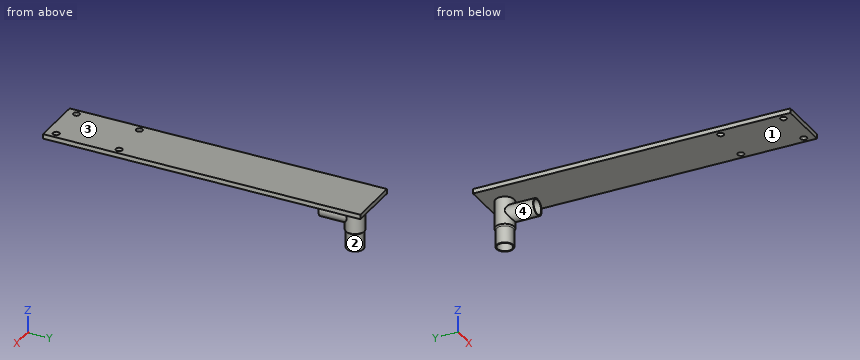
```python
from build123d import *

# Parameters (mm, degrees)
SKETCH_1_W             = 56
SKETCH_1_H             = 89.4
EXTRUDE_1_DEPTH        = 5
HOLE_WIZARD_M8_2_D     = 6.8
HOLE_WIZARD_M8_2_DEPTH = 19.75
HOLE_WIZARD_M8_2_TIP   = 2.042926105
SKETCH_7_W             = 56
SKETCH_7_H             = 5
EXTRUDE_2_DEPTH        = 252.5709
SKETCH_8_R             = 10
EXTRUDE_3_DEPTH        = 30
SKETCH_9_R             = 9
EXTRUDE_4_DEPTH        = 20
FILLET_1_R             = 2
EXTRUDE_START          = -20
SKETCH_10_R            = 9
EXTRUDE_5_DEPTH        = 35
SKETCH_11_R            = 8
CUT_EXTRUDE_1_DEPTH    = 40
SKETCH_12_R            = 8
CUT_EXTRUDE_2_DEPTH    = 45


with BuildPart() as part:
    # 草图1 → 凸台-拉伸1 (new body)
    with BuildSketch(Plane.XY):
        with Locations((28, -44.7)):
            Rectangle(SKETCH_1_W, SKETCH_1_H)
    extrude(amount=EXTRUDE_1_DEPTH)

    # M8 螺纹孔2
    with Locations(Plane.XY.offset(5)):
        with Locations((49.234030414, -78.598612839), (49.234030414, -10.801387161), (6.765969586, -10.801387161), (6.765969586, -78.598612839)):
            Hole(HOLE_WIZARD_M8_2_D / 2, depth=HOLE_WIZARD_M8_2_DEPTH)
            with Locations((0, 0, -(HOLE_WIZARD_M8_2_DEPTH + HOLE_WIZARD_M8_2_TIP / 2))):  # 118° drill point
                Cone(0, HOLE_WIZARD_M8_2_D / 2, HOLE_WIZARD_M8_2_TIP, mode=Mode.SUBTRACT)

    # 草图7 → 凸台-拉伸2 (add)
    with BuildSketch(Plane(origin=(0, 0, 0), x_dir=(1, 0, 0), z_dir=(0, 1, 0))):
        with Locations((28, -2.5)):
            Rectangle(SKETCH_7_W, SKETCH_7_H)
    extrude(amount=EXTRUDE_2_DEPTH)

    # 草图8 → 凸台-拉伸3 (add)
    with BuildSketch(Plane(origin=(0, 0, 0), x_dir=(-1, 0, 0), z_dir=(0, 0, -1))):
        with Locations(Location((-28, 232.5709, 0), (0, 0, 180))):
            Circle(SKETCH_8_R)
    extrude(amount=EXTRUDE_3_DEPTH)

    # 草图9 → 凸台-拉伸4 (add)
    with BuildSketch(Plane(origin=(0, 0, -30), x_dir=(-1, 0, 0), z_dir=(0, 0, -1))):
        with Locations((-28, 232.5709)):
            Circle(SKETCH_9_R)
    extrude(amount=EXTRUDE_4_DEPTH)

    # 圆角1
    # the kernel refuses this fillet: 2 mm, written as the material it adds along each edge
    with BuildSketch(Plane(origin=(28, 232.5709, -30), x_dir=(-1, 0, 0), z_dir=(0, -1, 0))) as fillet_1_piece_1:
        with BuildLine():
            CenterArc((11, 1.732050808), FILLET_1_R, 180, 60)
            Line((9, 1.732050808), (8.96, 1.732050808))
            Line((8.96, 1.732050808), (8.96, 0))
            Line((8.96, 0), (9, -0.04))
            ThreePointArc((9, -0.04), (9.5, -0.04), (9.98, -0.034641016))
            Line((9.98, -0.034641016), (10, 0))
        make_face()
    revolve(axis=Axis((28, 232.5709, -30), (0, 0, -1)))

    # 草图10 → 凸台-拉伸5 (add)
    with BuildSketch(Plane(origin=(0, 252.5709, 0), x_dir=(1, 0, 0), z_dir=(0, 1, 0)).offset(EXTRUDE_START)):
        with Locations(Location((28, 15, 0), (0, 0, 270))):
            Circle(SKETCH_10_R)
    extrude(amount=-EXTRUDE_5_DEPTH)

    # 草图11 → 切除-拉伸1 (cut)
    with BuildSketch(Plane.XZ.offset(-197.5709)):
        with Locations(Location((28, -15, 0), (0, 0, 270))):
            Circle(SKETCH_11_R)
    extrude(amount=-CUT_EXTRUDE_1_DEPTH, mode=Mode.SUBTRACT)

    # 草图12 → 切除-拉伸2 (cut)
    with BuildSketch(Plane(origin=(0, 0, -50), x_dir=(-1, 0, 0), z_dir=(0, 0, -1))):
        with Locations((-28, 232.5709)):
            Circle(SKETCH_12_R)
    extrude(amount=-CUT_EXTRUDE_2_DEPTH, mode=Mode.SUBTRACT)


solid = part.part
```
Design review of the part built by this model. Coordinates are the model's own, in mm. Face numbers are marked on the shaded views. A direction names the side the tool comes from. Give positions to 0.01 mm unless a question says otherwise; leave off trailing zeros. Loops run counter-clockwise (first coordinate to the right, second up) from the corner with the lowest first, then second, coordinate; pieces in that order, holes last. Notation, with made-up numbers: M -29,42.25 L 12,42.25 A19 cw 12,64.25 Z; hole C 8.25,-2.75 d11. An arc over 180 degrees is marked long. Return JSON: item names as keys, results as strings. Group by question number.
Item 1: We need section B-B (z = -42). Give the boundary of the cut face in (x, y).
Item 2: Insertion check: pin 1 Ø5 at (x, y) = (20.5, 216.5) entering from -Z; pin 2 Ø9.5 at (x, z) = (28, -15) entering from -Y; pin 3 Ø2 at (x, y) = (8, 125.5) entering from -Z. Each pin has a flat end and moves straight along its axis. Give the tip position at first contact, or say it passes through.
Item 3: We need section C-C (y = -19). Give the boundary of the cut face in (x, z), and give its area (3 significant figures).
Item 4: We need section A-A (x = 28). Give the boundary of the cut face in (y, z).
Item 5: Tool access review of the marked faces 3 and 4: name each direction out of +Z, -Z, +X, -X, +Y, -Y from which nothing blocks a thin tool from reaching the whole face with its end or side.
Item 6: For probe 1 along Z at (x, y) = (28, 217); probe 2 along Y at (x, z) = (27, -25.5); probe 3 along Z at (x, y) = (15.5, -37.5), list the stretches that pass through material, from the lowest coordinate up.
Item 7: Mouldability with a two-part tool opening along Y and no side actions: class the marked faces 1 and 2 as released by +Y, released by -Y, zero draft, split by the parting line, or undercut.
Item 8: We need section D-D (x = 41). Give the boundary of the cut face in (y, z), and give its area (3 significant figures).
Output:
{
 "1": {"outline": "C 28,232.57 d18; hole C 28,232.57 d16"},
 "2": {"pin 1": "stops at z = -22.48", "pin 2": "stops at y = 239.01", "pin 3": "stops at z = 0"},
 "3": {"outline": "M 0,0 L 56,0 L 56,5 L 0,5 Z", "area": "280 mm^2"},
 "4": {"outline": "M -89.4,0 L 222.57,0 L 222.57,-6 L 197.57,-6 L 197.57,-7 L 224.57,-7 L 224.57,-5 L 240.57,-5 L 240.57,-50 L 241.57,-50 L 241.57,-31.73 A2 cw 242.57,-30 L 242.57,0 L 252.57,0 L 252.57,5 L -89.4,5 Z; M 197.57,-24 L 222.57,-24 L 222.57,-30 A2 cw 223.57,-31.73 L 223.57,-50 L 224.57,-50 L 224.57,-23 L 197.57,-23 Z"},
 "5": {"face 3": "+Z, +X, -X, +Y, -Y", "face 4": "-Y"},
 "6": {"probe 1": "z = -24 to -23, -7 to -6, 0 to 5", "probe 2": "y = 222.62 to 224.63, 240.51 to 242.52", "probe 3": "z = 0 to 5"},
 "7": {"face 1": "zero draft", "face 2": "split by the parting line"},
 "8": {"outline": "M -89.4,0 L 252.57,0 L 252.57,5 L -89.4,5 Z", "area": "1,710 mm^2"}
}
